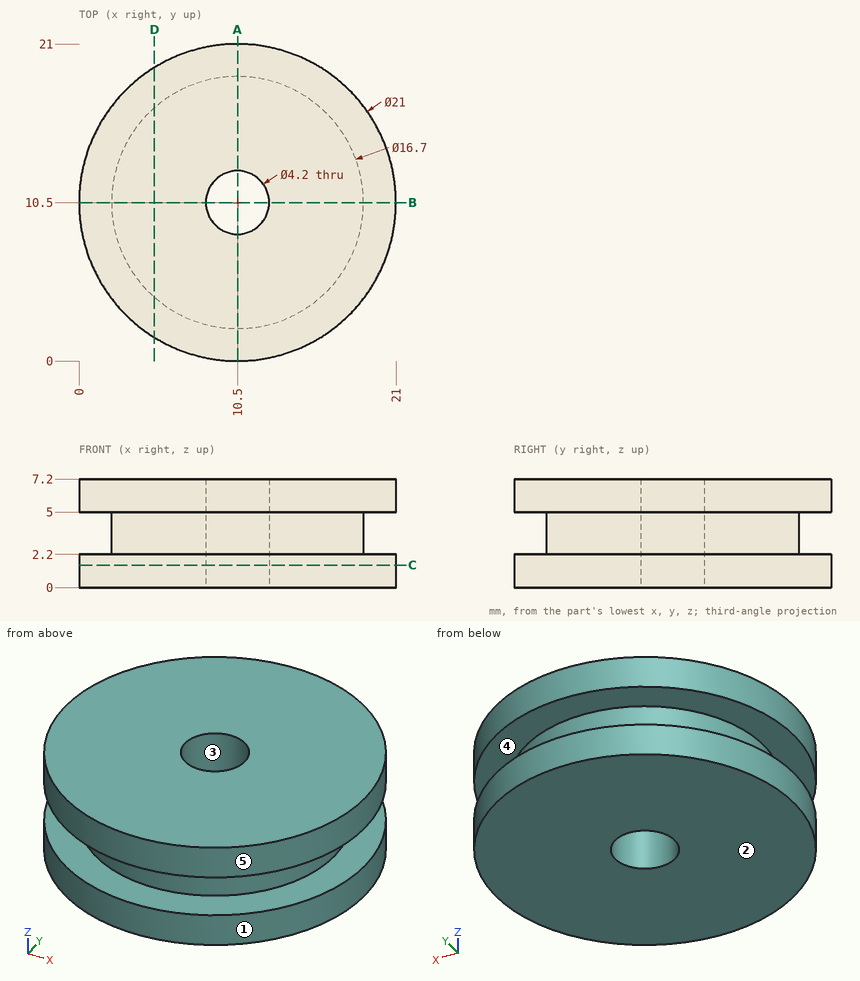
The figure shows three views and two pictorial views of one solid part (mm, origin at its lowest corner). Answer the questions. A direction names the side the tool comes from. Coordinates: 2 decimals unless noted, no trailing zeros. Loops run counter-clockwise (first coordinate to the right, second up) from the corner with the lowest first, then second, coordinate; pieces in that order, holes last. Notation, with made-up numbers: M 56,61.25 L 65,61.25 A27 cw 65,85.25 Z; hole C -5.75,32 d1. An arc over 180 degrees is marked long. Answer as CSV lines item,"result". Start each with the question number.
(1) The part is cut by section C-C (z = 1.5). Give the vertices of the cut face in (x, y).
(2) Given pin 1 (3 mm diameter, centred on y = 13, z = 1, fed in from +X); pin 2 (1 mm diameter, centred on y = 3.5, z = 1.5, fed in from +X); pin 3 (1.5 mm diameter, centred on x = 3.5, z = 1.5, fed in from -Y), each flat-ended and moving along its own axis, determine where each tip first touches the part or whether it passes through.
(3) The part is cut by section A-A (x = 10.5). Give the vertices of the cut face in (y, z), and give its area (3 significant figures).
(4) The part is cut by section D-D (x = 5). Give the vertices of the cut face in (y, z).
(5) Find the intervals of material crossed by L1, parallel to Y at x = 10.5, z = 5.25; L2, parallel to Y at x = 10.5, z = 3.25; L3, parallel to Z at x = 5.25, y = 1.75, in increasing order. Write a range as [from, to].
(6) For the marked faces 4 and 5, determine the directions among +Z, -Z, +X, -X, +Y, -Y from which every point of the face is accessible in a straight line to the end or side of a thin tool.
(7) The mould has two halves that part along X. Classify the marked faces 1, 2 and 3: pulls with the +X half, pulls with the -X half, needs draft (parallel to the pull), parting line crosses it, or undercut.
Determined:
1,outline,"C 10.5,10.5 d21; hole C 10.5,10.5 d4.2"
2,pin 1,"x = 20.95"
2,pin 2,"x = 18.75"
2,pin 3,"y = 2.06"
3,outline,"M 0,0 L 8.4,0 L 8.4,7.2 L 0,7.2 L 0,5 L 2.15,5 L 2.15,2.2 L 0,2.2 Z; M 12.6,0 L 21,0 L 21,2.2 L 18.85,2.2 L 18.85,5 L 21,5 L 21,7.2 L 12.6,7.2 Z"
3,area,"109 mm2"
4,outline,"M 1.56,0 L 19.44,0 L 19.44,2.2 L 16.78,2.2 L 16.78,5 L 19.44,5 L 19.44,7.2 L 1.56,7.2 L 1.56,5 L 4.22,5 L 4.22,2.2 L 1.56,2.2 Z"
5,L1,"[0, 8.4], [12.6, 21]"
5,L2,"[2.15, 8.4], [12.6, 18.85]"
5,L3,"[0, 2.2], [5, 7.2]"
6,face 4,"none"
6,face 5,"+Z, -Z"
7,face 1,"parting line crosses it"
7,face 2,"needs draft"
7,face 3,"undercut"
